Design review of the part shown in the three views and the two pictorial views. Dimensions are in mm from the part's minimum x, y and z. Give positions to 0.01 mm unless a question says otherwise; leave off trailing zeros. Loops run counter-clockwise (first coordinate to the right, second up) from the corner with the lowest first, then second, coordinate; pieces in that order, holes last. Notation, with made-up numbers: (39.5, 72) -> (51.5, 72) arc R25 ccw to (51.5, 89) -> close; hole circle Ø4 at (23, 70.25). An arc over 180 degrees is marked (long way). Use CSV: the item, a comma, the result in double quotes. Start each with the question number.
Item 1: We need section D-D (y = 13). State the section outline as (x, z) points.
Item 2: We need section A-A (y = 59). State the section outline as (x, z) points.
Item 3: We need section B-B (x = 28). State the section outline as (y, z) points, plus the area to 3 significant figures.
Item 4: Clearance check with flat-ended pins moving along their axes: pin 1 (0.9 mm diameter, centred on x = 24.5, z = 1, fed in from +Y); pin 2 (1.5 mm diameter, centred on y = 1, z = 1.5, fed in from -X); pin 3 (1.5 mm diameter, centred on y = 1.5, z = 1.5, fed in from +X). State where each tip first meets the part, or that it passes through.
Item 5: Wall thickness on line 1 along X through (y, z) = (94, 1.5); line 2 along Y through (x, z) = (88, 2.3); line 3 along Y through (x, z) = (53.5, 1.6): over which ranges is each line inside the solid? List them lowest first. Write a range as from..to.
Item 6: We need section C-C (z = 0.65). Count the separate pieces of the cut face and the enclosed holes in it, plus the area to 3 significant figures.
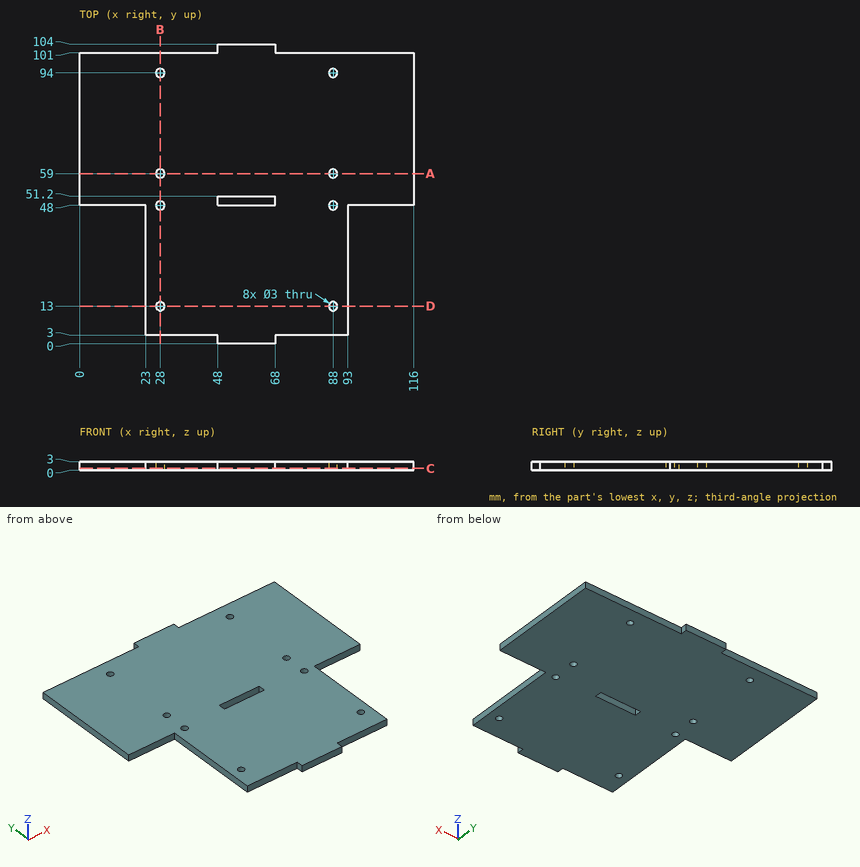
Results found:
1,outline,"(23, 0) -> (26.5, 0) -> (26.5, 3) -> (23, 3) -> close; (29.5, 0) -> (86.5, 0) -> (86.5, 3) -> (29.5, 3) -> close; (89.5, 0) -> (93, 0) -> (93, 3) -> (89.5, 3) -> close"
2,outline,"(0, 0) -> (26.5, 0) -> (26.5, 3) -> (0, 3) -> close; (29.5, 0) -> (86.5, 0) -> (86.5, 3) -> (29.5, 3) -> close; (89.5, 0) -> (116, 0) -> (116, 3) -> (89.5, 3) -> close"
3,outline,"(3, 0) -> (11.5, 0) -> (11.5, 3) -> (3, 3) -> close; (14.5, 0) -> (46.5, 0) -> (46.5, 3) -> (14.5, 3) -> close; (49.5, 0) -> (57.5, 0) -> (57.5, 3) -> (49.5, 3) -> close; (60.5, 0) -> (92.5, 0) -> (92.5, 3) -> (60.5, 3) -> close; (95.5, 0) -> (101, 0) -> (101, 3) -> (95.5, 3) -> close"
3,area,"258 mm²"
4,pin 1,"y = 101"
4,pin 2,"x = 48"
4,pin 3,"x = 68"
5,line 1,"0..26.5, 29.5..86.5, 89.5..116"
5,line 2,"3..11.5, 14.5..46.5, 49.5..57.5, 60.5..92.5, 95.5..101"
5,line 3,"0..48, 51.2..104"
6,separate pieces,"1"
6,enclosed holes,"9"
6,area,"9,300 mm²"
